Check sheet for the modelled part. Datum: model origin and axes. Units: mm. Face numbers are marked on the shaded views. Give positions to 0.01 mm unless a question says otherwise; leave off trailing zeros.
```python
from build123d import *

# Parameters (mm, degrees)
EXTRUDE_1_DEPTH     = 3
CUT_EXTRUDE_4_DEPTH = 10
SKETCH_6_W          = 3
SKETCH_6_H          = 0.29
EXTRUDE_4_DEPTH     = 3


with BuildPart() as part:
    # 草图1 → 凸台-拉伸1 (new body)
    with BuildSketch(Plane.XY):
        with BuildLine():
            Line((-64.999999986, 52.296752884), (-60.705196958, 52.296752884))
            Line((-60.705196958, 52.296752884), (-60.705196958, 55.296750271))
            Line((-60.705196958, 55.296750271), (-45.705196958, 55.296750271))
            Line((-45.705196958, 55.296750271), (-45.705196958, 52.296752929))
            Line((-45.705196958, 52.296752929), (-42.249528739, 52.296752929))
            add(Edge.make_bspline(
                [(-42.249528739, 52.296752929), (0, -12.296752929), (42.249528739, 52.296752929)],
                knots=[0, 0, 0, 1, 1, 1], degree=2))
            Line((42.249528739, 52.296752929), (45.705196958, 52.296752929))
            Line((45.705196958, 52.296752929), (45.705196958, 55.296750271))
            Line((45.705196958, 55.296750271), (60.705196958, 55.296750271))
            Line((60.705196958, 55.296750271), (60.705196958, 52.296752884))
            Line((60.705196958, 52.296752884), (64.999999986, 52.296752884))
            add(Edge.make_bspline(
                [(-64.999999986, 52.296752884), (-32.499999991, -52.296752885), (0, 52.296752883), (32.499999995, -52.296752882), (64.999999986, 52.296752884)],
                knots=[0.035680117, 0.035680117, 0.035680117, 0.035680117, 0.035680117, 0.964319883, 0.964319883, 0.964319883, 0.964319883, 0.964319883], degree=4))
        make_face()
    extrude(amount=EXTRUDE_1_DEPTH)

    # 草图4 → 切除-拉伸4 (cut)
    with BuildSketch(Plane.XY.offset(3)):
        Polygon((-1.5, 1.4832e-05), (-1.5, -2.686062371), (1.5, -2.686062371), (1.5, 0.000504044), (1.5, 10.2), (-1.5, 10.2), align=None)
    extrude(amount=-CUT_EXTRUDE_4_DEPTH, mode=Mode.SUBTRACT)

    # 草图6 → 凸台-拉伸4 (add)
    with BuildSketch(Plane(origin=(0, 0, 0), x_dir=(-1, 0, 0), z_dir=(0, 0, -1))):
        with Locations((0, 10.055)):
            Rectangle(SKETCH_6_W, SKETCH_6_H)
    extrude(amount=-EXTRUDE_4_DEPTH)


solid = part.part
```
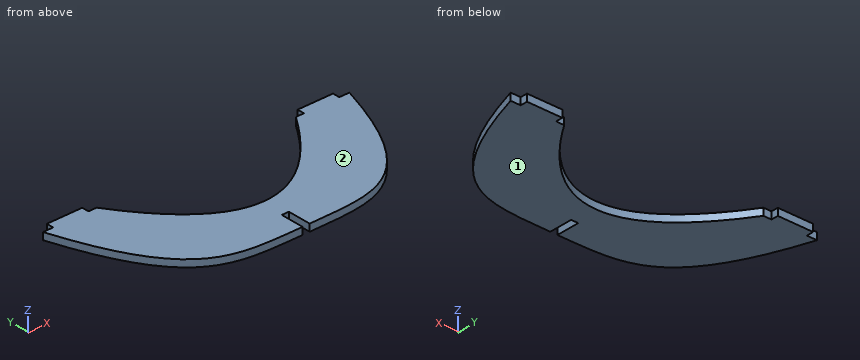
(1) Thickness scan on L1, parallel to X at y = 30.5, z = 2.6; L2, parallel to X at y = 52.5, z = 1; L3, parallel to Y at x = 17.5, z = 0.45. Record the ranges inside material, lowest first.
(2) Go/stop test with flat-tipped pins: P1, Ø1.5, axis at x = 64, z = 1.5, coming from the +Y side; P2, Ø0.9, axis at y = 4.5, z = 2, coming from the -X side; P3, Ø0.9, axis at y = 53.5, z = 1, coming from the +X side. Record where each tip stops, or that it passes through.
(3) Release check for a two-part mould opening along Z. For the marked faces 1 and 2 record: released by +Z, released by -Z, zero draft, split by the parting line, or undercut.
Values follow:
1. L1: x = -56.8 to -24.09, 24.09 to 56.8
1. L2: x = -60.71 to -45.71, 45.71 to 60.71
1. L3: y = 0.27 to 25.54
2. P1: stops at y = 52.3
2. P2: stops at x = -36.05
2. P3: stops at x = 60.71
3. face 1: released by -Z
3. face 2: released by +Z
